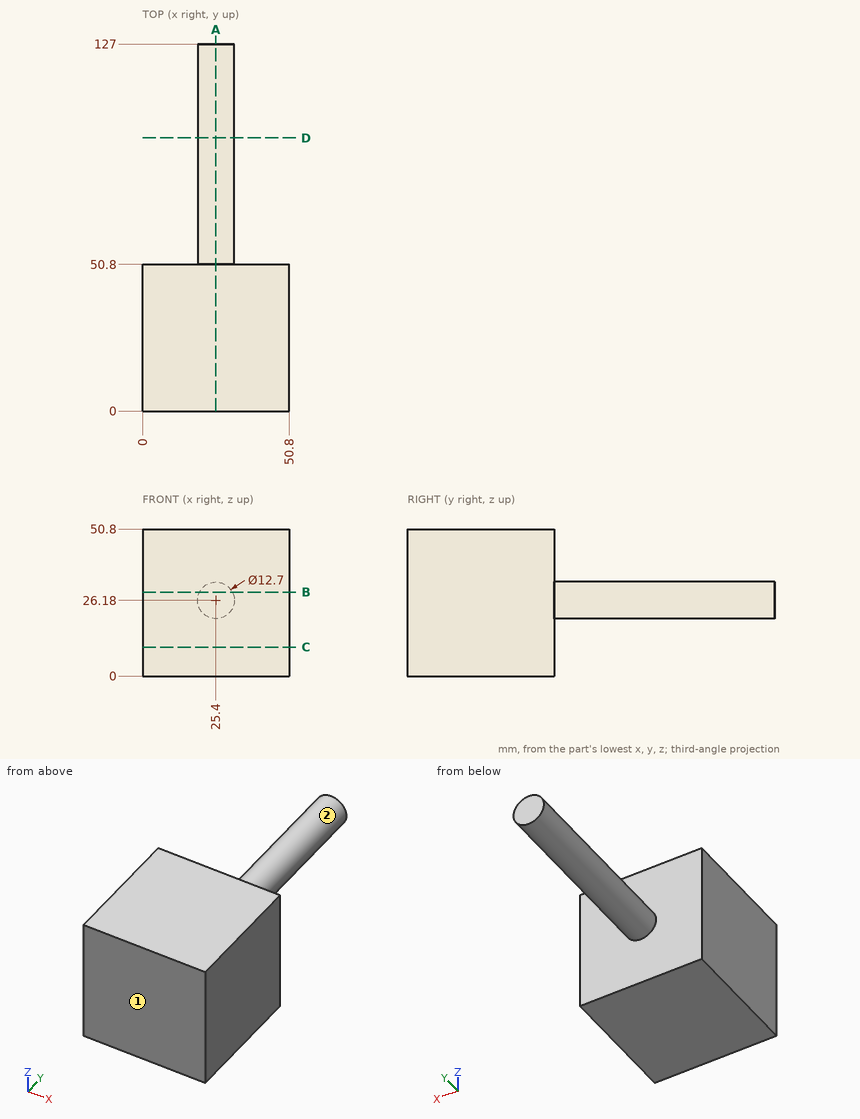
Answer from the drawing. Dimensions are ordinates in mm from the lowest x, y and z of the part. A direction names the side the tool comes from. Round coordinates to 2 decimals unless told otherwise and drop trailing zeros. Loops run counter-clockwise (first coordinate to the right, second up) from the corner with the lowest first, then second, coordinate; pieces in that order, holes last.
1) For the marked faces 1 and 2, determine the directions among +Z, -Z, +X, -X, +Y, -Y from which every point of the face is accessible in a straight line to the end or side of a thin tool.
Outcome:
face 1: +Z, -Z, +X, -X, -Y
face 2: +Y
2) A cutting plane is placed at B-B on z = 29. Determine the outline of the cut face in (x, y), plus the area to 3 significant figures.
Outcome:
outline: (0, 0) - (50.8, 0) - (50.8, 50.8) - (31.09, 50.8) - (31.09, 127) - (19.71, 127) - (19.71, 50.8) - (0, 50.8) - close
area: 3,450 mm2
3) Given P1, Ø10, axis at x = 44.5, z = 11.5, coming from the +Y side; P2, Ø4, axis at x = 38, z = 19, coming from the -Y side; P3, Ø3, axis at x = 20, y = 110, coming from the -Z side; P4, Ø10, axis at y = 60.5, z = 24.5, coming from the -X side, each flat-ended and moving along its own axis, determine where each tip first touches the part or whether it passes through.
Outcome:
P1: stops at y = 50.8
P2: stops at y = 0
P3: stops at z = 21.17
P4: stops at x = 19.05
4) Consider line 1 (Y direction, x = 48, z = 38.5); line 2 (X direction, y = 59.5, z = 26); line 3 (Z direction, x = 21, y = 109). Determine where each line is inside the solid, lowest interval first.
Outcome:
line 1: y = 0 to 50.8
line 2: x = 19.05 to 31.75
line 3: z = 21.6 to 30.76
5) A cutting plane is placed at D-D on y = 94.5. Determine the outline of the cut face in (x, z), plus the area to 3 significant figures.
Outcome:
outline: circle Ø12.7 at (25.4, 26.18)
area: 127 mm2
6) A cutting plane is placed at C-C on z = 10. Determine the outline of the cut face in (x, y), plus the area to 3 significant figures.
Outcome:
outline: (0, 0) - (50.8, 0) - (50.8, 50.8) - (0, 50.8) - close
area: 2,580 mm2
7) A cutting plane is placed at A-A on x = 25.4. Determine the outline of the cut face in (y, z).
Outcome:
outline: (0, 0) - (50.8, 0) - (50.8, 19.83) - (127, 19.83) - (127, 32.53) - (50.8, 32.53) - (50.8, 50.8) - (0, 50.8) - close
